Design review of the part built by this model. Coordinates are the model's own, in mm. A direction names the side the tool comes from. Coordinates: 2 decimals unless noted, no trailing zeros. Write each loop counter-clockwise with the first axis right and the second up, starting at its lowest first coordinate (ties: lowest second). Pieces come first, ordered by that corner, then holes. Notation, with made-up numbers: (82.25, 42.5) - (120.25, 42.5) arc R36 cw to (120.25, 76.5) - close; hole circle Ø2 at (22.25, 11.5). An arc over 180 degrees is marked (long way). Use a Markdown table: item, result.
from build123d import *

# Parameters (mm, degrees)
BOSS_EXTRUDE1_DEPTH = 2.2
BOSS_EXTRUDE2_DEPTH = 2
FILLET1_R           = 0.5
FILLET2_R           = 3


with BuildPart() as part:
    # Sketch3 → Boss-Extrude1 (new body)
    with BuildSketch(Plane.XY):
        with BuildLine():
            ThreePointArc((-7.35, 0), (-7.238336985, 1.276314106), (-6.906740763, 2.513848053))
            Line((-6.906740763, 2.513848053), (-8.551202849, 3.112383304))
            ThreePointArc((-8.551202849, 3.112383304), (-8.961750552, 1.580198417), (-9.1, 0))
            Line((-9.1, 0), (-7.35, 0))
        make_face()
        with BuildLine():
            Line((-8.551202849, 3.112383304), (-6.906740763, 2.513848053))
            ThreePointArc((-6.906740763, 2.513848053), (-4.474396503, 5.831147051), (-0.640594709, 7.322031031))
            Line((-0.640594709, 7.322031031), (-0.793117259, 9.065371753))
            ThreePointArc((-0.793117259, 9.065371753), (-5.539729004, 7.219515397), (-8.551202849, 3.112383304))
        make_face()
        with BuildLine():
            Line((3.550704156, 6.15), (7.101408311, 0))
            Line((7.101408311, 0), (7.35, 0))
            ThreePointArc((7.35, 0), (4.965588026, 5.418988426), (-0.640594709, 7.322031031))
            Line((-0.640594709, 7.322031031), (-0.538055281, 6.15))
            Line((-0.538055281, 6.15), (3.550704156, 6.15))
        make_face()
        with BuildLine():
            ThreePointArc((-0.501145521, 5.728119514), (3.884643694, 4.239344687), (5.75, 0))
            Line((5.75, 0), (7.101408311, 0))
            Line((7.101408311, 0), (3.550704156, 6.15))
            Line((3.550704156, 6.15), (-0.538055281, 6.15))
            Line((-0.538055281, 6.15), (-0.501145521, 5.728119514))
        make_face()
        with BuildLine():
            Line((-5.868261699, 2.135872585), (-5.40323257, 1.966615824))
            ThreePointArc((-5.40323257, 1.966615824), (-3.500378217, 4.561781707), (-0.501145521, 5.728119514))
            Line((-0.501145521, 5.728119514), (-0.538055281, 6.15))
            Line((-0.538055281, 6.15), (-3.550704156, 6.15))
            Line((-3.550704156, 6.15), (-5.868261699, 2.135872585))
        make_face()
        with BuildLine():
            Line((-6.906740763, 2.513848053), (-5.868261699, 2.135872585))
            Line((-5.868261699, 2.135872585), (-3.550704156, 6.15))
            Line((-3.550704156, 6.15), (-0.538055281, 6.15))
            Line((-0.538055281, 6.15), (-0.640594709, 7.322031031))
            ThreePointArc((-0.640594709, 7.322031031), (-4.474396503, 5.831147051), (-6.906740763, 2.513848053))
        make_face()
        with BuildLine():
            Line((-7.101408311, 0), (-5.868261699, 2.135872585))
            Line((-5.868261699, 2.135872585), (-6.906740763, 2.513848053))
            ThreePointArc((-6.906740763, 2.513848053), (-7.238336985, 1.276314106), (-7.35, 0))
            Line((-7.35, 0), (-7.101408311, 0))
        make_face()
        with BuildLine():
            ThreePointArc((-5.75, 0), (-5.66264458, 0.998477022), (-5.40323257, 1.966615824))
            Line((-5.40323257, 1.966615824), (-5.868261699, 2.135872585))
            Line((-5.868261699, 2.135872585), (-7.101408311, 0))
            Line((-7.101408311, 0), (-5.75, 0))
        make_face()
        with BuildLine():
            Line((7.101408311, 0), (5.868261699, -2.135872585))
            Line((5.868261699, -2.135872585), (6.906740763, -2.513848053))
            ThreePointArc((6.906740763, -2.513848053), (7.238336985, -1.276314106), (7.35, 0))
            Line((7.35, 0), (7.101408311, 0))
        make_face()
        with BuildLine():
            ThreePointArc((5.75, 0), (5.66264458, -0.998477022), (5.40323257, -1.966615824))
            Line((5.40323257, -1.966615824), (5.868261699, -2.135872585))
            Line((5.868261699, -2.135872585), (7.101408311, 0))
            Line((7.101408311, 0), (5.75, 0))
        make_face()
        with BuildLine():
            Line((6.906740763, -2.513848053), (5.868261699, -2.135872585))
            Line((5.868261699, -2.135872585), (3.550704156, -6.15))
            Line((3.550704156, -6.15), (0.538055281, -6.15))
            Line((0.538055281, -6.15), (0.640594709, -7.322031031))
            ThreePointArc((0.640594709, -7.322031031), (4.474396503, -5.831147051), (6.906740763, -2.513848053))
        make_face()
        with BuildLine():
            Line((5.868261699, -2.135872585), (5.40323257, -1.966615824))
            ThreePointArc((5.40323257, -1.966615824), (3.500378217, -4.561781707), (0.501145521, -5.728119514))
            Line((0.501145521, -5.728119514), (0.538055281, -6.15))
            Line((0.538055281, -6.15), (3.550704156, -6.15))
            Line((3.550704156, -6.15), (5.868261699, -2.135872585))
        make_face()
        with BuildLine():
            Line((-3.550704156, -6.15), (-7.101408311, 0))
            Line((-7.101408311, 0), (-7.35, 0))
            ThreePointArc((-7.35, 0), (-4.965588026, -5.418988426), (0.640594709, -7.322031031))
            Line((0.640594709, -7.322031031), (0.538055281, -6.15))
            Line((0.538055281, -6.15), (-3.550704156, -6.15))
        make_face()
        with BuildLine():
            ThreePointArc((0.501145521, -5.728119514), (-3.884643694, -4.239344687), (-5.75, 0))
            Line((-5.75, 0), (-7.101408311, 0))
            Line((-7.101408311, 0), (-3.550704156, -6.15))
            Line((-3.550704156, -6.15), (0.538055281, -6.15))
            Line((0.538055281, -6.15), (0.501145521, -5.728119514))
        make_face()
        with BuildLine():
            Line((8.551202849, -3.112383304), (6.906740763, -2.513848053))
            ThreePointArc((6.906740763, -2.513848053), (4.474396503, -5.831147051), (0.640594709, -7.322031031))
            Line((0.640594709, -7.322031031), (0.793117259, -9.065371753))
            ThreePointArc((0.793117259, -9.065371753), (5.539729004, -7.219515397), (8.551202849, -3.112383304))
        make_face()
        with BuildLine():
            ThreePointArc((7.35, 0), (7.238336985, -1.276314106), (6.906740763, -2.513848053))
            Line((6.906740763, -2.513848053), (8.551202849, -3.112383304))
            ThreePointArc((8.551202849, -3.112383304), (8.961750552, -1.580198417), (9.1, 0))
            Line((9.1, 0), (7.35, 0))
        make_face()
    extrude(amount=BOSS_EXTRUDE1_DEPTH)

    # Sketch4 → Boss-Extrude2 (add)
    with BuildSketch(Plane.XY.offset(2.2)):
        with BuildLine():
            Line((-7.35, 0), (-5.75, 0))
            ThreePointArc((-5.75, 0), (-5.66264458, 0.998477022), (-5.40323257, 1.966615824))
            Line((-5.40323257, 1.966615824), (-8.551202849, 3.112383304))
            ThreePointArc((-8.551202849, 3.112383304), (-8.961750552, 1.580198417), (-9.1, 0))
            Line((-9.1, 0), (-7.35, 0))
        make_face()
        with BuildLine():
            Line((7.35, 0), (5.75, 0))
            ThreePointArc((5.75, 0), (5.66264458, -0.998477022), (5.40323257, -1.966615824))
            Line((5.40323257, -1.966615824), (8.551202849, -3.112383304))
            ThreePointArc((8.551202849, -3.112383304), (8.961750552, -1.580198417), (9.1, 0))
            Line((9.1, 0), (7.35, 0))
        make_face()
    extrude(amount=BOSS_EXTRUDE2_DEPTH)

    # Fillet1
    fillet1_edges = [part.edges().sort_by_distance(p)[0] for p in [
        (-5.66264458, 0.998477022, 4.2),
        (-6.977217709, 2.539499564, 4.2),
        (-8.961750552, 1.580198417, 4.2),
        (-7.425, 0, 4.2),
        (5.66264458, -0.998477022, 4.2),
        (6.977217709, -2.539499564, 4.2),
        (8.961750552, -1.580198417, 4.2),
        (7.425, 0, 4.2),
    ]]
    fillet(fillet1_edges, radius=FILLET1_R)

    # Fillet2
    # the kernel refuses this fillet: 3 mm, written as the material it takes off along each edge
    with BuildSketch(Plane(origin=(0.010596731, -0.121121189, 2.2), x_dir=(0.9961946980917455, 0.08715574274765829, 0), z_dir=(0.0871557427476583, -0.9961946980917455, 0))) as fillet2_piece_1_section:
        with BuildLine():
            CenterArc((2.891366459, -3), FILLET2_R, 90, 74.533990047)
            Line((0, -2.2), (0, 0))
            Line((0, 0), (2.891366459, 0))
        make_face()
    fillet2_piece_1 = extrude(amount=16.206832295, mode=Mode.PRIVATE)
    fillet2_piece_1 = fillet2_piece_1 - Plane(origin=(0, 0, 1.592242212), x_dir=(1, 0, 0), z_dir=(0, 0, -1)) * Cylinder(7.35, 44, mode=Mode.PRIVATE)
    add(fillet2_piece_1, mode=Mode.SUBTRACT)
    with BuildSketch(Plane(origin=(-0.010596731, 0.121121189, 2.2), x_dir=(-0.9961946980917455, -0.08715574274765826, 0), z_dir=(-0.08715574274765826, 0.9961946980917455, 0))) as fillet2_piece_2_section:
        with BuildLine():
            CenterArc((2.891366459, -3), FILLET2_R, 90, 74.533990047)
            Line((0, -2.2), (0, 0))
            Line((0, 0), (2.891366459, 0))
        make_face()
    fillet2_piece_2 = extrude(amount=16.206832295, mode=Mode.PRIVATE)
    fillet2_piece_2 = fillet2_piece_2 - Plane(origin=(0, 0, 1.592242212), x_dir=(1, 0, 0), z_dir=(0, 0, -1)) * Cylinder(7.35, 44, mode=Mode.PRIVATE)
    add(fillet2_piece_2, mode=Mode.SUBTRACT)


solid = part.part
(1) For pin 1 (4 mm diameter, centred on x = -4, y = -7, fed in from +Z); pin 2 (1 mm diameter, centred on x = -7, z = 1, fed in from -Y); pin 3 (1.5 mm diameter, centred on x = -6, z = 1, fed in from -Y), all flat-tipped, find the tip position at first contact; note any pin that passes through.
Determined:
| item | result |
|---|---|
| pin 1 | z = 2.2 |
| pin 2 | y = -3.43 |
| pin 3 | y = -5.14 |
(2) For L1, parallel to Y at x = 0, z = 1.6; L2, parallel to Y at x = -2.75, z = 0.7; L3, parallel to Z at x = 4.25, y = -6.25, list the stretches that pass through material, from the lowest coordinate up. Write a range as from..to.
Determined:
| item | result |
|---|---|
| L1 | -7.35..-5.75, 5.75..7.35 |
| L2 | -6.82..-5.05, 5.05..8.67 |
| L3 | 0..2.2 |
(3) Take a section at B-B on z = 3.05. Write out the cut boundary in (x, y).
Determined:
| item | result |
|---|---|
| outline | (-9.1, 0) - (-5.75, 0) arc R5.75 cw to (-5.4, 1.97) - (-8.55, 3.11) arc R9.1 ccw to start; (5.4, -1.97) - (8.55, -3.11) arc R9.1 ccw to (9.1, 0) - (5.75, 0) arc R5.75 cw to start |
(4) Machinability: for faces 4 (the cylindrical face through (1.8, -8.05, 1.6)), 5 (the cylindrical face through (-1.8, 8.05, 1.6)), 6 (the flat face through (-8, 0, 2)), 7 (the cylindrical face through (-7.575, 5.043, 1.413)), 8 (the flat face through (8, 0, 2)), which of the approach directions +Z, -Z, +X, -X, +Y, -Y give a long, thin tool a straight path to every point of the face, cutting with its end or side? Answer none if there is none.
Determined:
| item | result |
|---|---|
| face 4 | +Z, -Y |
| face 5 | +Z, +Y |
| face 6 | +Z, -X, -Y |
| face 7 | +Z, -Z, -X, +Y |
| face 8 | +Z, +X, +Y |
(5) Take a section at C-C on y = 6.25. Write out the cut boundary in (x, z), and give its area (3 significant figures).
Determined:
| item | result |
|---|---|
| outline | (-6.61, 0) - (3.87, 0) - (3.87, 2.2) - (-6.61, 2.2) - close |
| area | 23.1 mm2 |
(6) Take a section at A-A on x = 0. Write out the cut boundary in (y, z), and give its area (3 significant figures).
Determined:
| item | result |
|---|---|
| outline | (-7.35, 0) - (-5.75, 0) - (-5.75, 2.2) - (-7.35, 2.2) - close; (5.75, 0) - (7.35, 0) - (7.35, 2.2) - (5.75, 2.2) - close |
| area | 7.04 mm2 |
(7) Draft analysis for pull direction Y (two halves, no side actions). For faces 1 (the flat face through (-6.955, 2.531, 2.94)), 2 (the cylindrical face through (-5.484, 1.727, 1.002)), 3 (the flat face through (7, -1, 4.2)), state which applies: +Y half, -Y half, draft (parallel to the pull), parting line (faces both ways), or undercut.
Determined:
| item | result |
|---|---|
| face 1 | +Y half |
| face 2 | undercut |
| face 3 | draft |
